Geometry check sheet. Reference: the model listing, model coordinates, mm. A direction names the side the tool comes from. Coordinates: 2 decimals unless noted, no trailing zeros. Write each loop counter-clockwise with the first axis right and the second up, starting at its lowest first coordinate (ties: lowest second). Pieces come first, ordered by that corner, then holes. Notation, with made-up numbers: (-15.5, 70) -> (42.5, 70) arc R10 ccw to (42.5, 86) -> close; hole circle Ø3 at (-2.5, 54). An arc over 180 degrees is marked (long way). Answer in a Markdown table with one row per item. Add a question column.
1. Cross-section at C-C on x = -197. Record the cut outline in (y, z).
2. Cross-section at A-A on y = 122.5. Record the cut outline in (x, z), and give its area (3 significant figures).
3. Cross-section at D-D on x = 57. Record the cut outline in (y, z).
4. Cross-section at B-B on z = 27.5. Record the cut outline in (x, y).
5. Depth check by flat-ended pin: P1, Ø1, axis at x = 134, z = 7, coming from the +Y side; P2, Ø3, axis at x = 190.5, z = 4.5, coming from the +Y side. Enter the tip coordinate at first touch or a pass-through.
6. Mould release check, pull along X, two halves, no side actions. Record for faces 1 (the flat face through (256.851, 121, 19)), 2 (the flat face through (153.663, 242, 19)), 3 (the flat face through (49, 66, 38.1)): pulls with the +X half, pulls with the -X half, needs draft (parallel to the pull), parting line crosses it, or undercut.
7. Scan lines: L1, parallel to X at y = 281.5, z = 8; L2, parallel to Z at x = -175.5, y = 334; L3, parallel to Y at x = 118, z = 34. Record each from-to range of solid material in increasing order. Write a range as from..to.
8. Set-up check for faces 4 (the flat face through (92, 79.238, 19)), 5 (the flat face through (205, 348, 6.35)), 6 (the cylindrical face through (-6.059, 31.626, 19.317)): record each of +Z, -Z, +X, -X, +Y, -Y from which the full face is reachable in a straight line by a thin tool's end or side.
```python
from build123d import *

# Parameters (mm, degrees)
F0_W     = 523.875
F0_H     = 568.325
F1_DEPTH = 38.1
F2_R     = 38.1
F3_DEPTH = 50.8
F4_W     = 317.5
F4_H     = 330.2
F5_DEPTH = 50.8
F6_W     = 896.055773
F6_H     = 120.65
F7_DEPTH = 6.35


with BuildPart() as f1:
    # F0 (on Top) → F1 (new body)
    with BuildSketch(Plane.XY):
        with Locations((-5.086774, 125.275676)):
            Rectangle(F0_W, F0_H)
    extrude(amount=F1_DEPTH)

    # F2 (on face) → F3 (cut)
    with BuildSketch(Plane.XY.offset(38.1)):
        with Locations((-5.086774, 69.713176)):
            Circle(F2_R)
    extrude(amount=-F3_DEPTH, mode=Mode.SUBTRACT)

    # F4 (on face) → F5 (cut)
    with BuildSketch(Plane.XY.offset(38.1)):
        with Locations((-5.086774, 244.338176)):
            Rectangle(F4_W, F4_H)
    extrude(amount=-F5_DEPTH, mode=Mode.SUBTRACT)

    # F6 (on face) → F7 (cut)
    with BuildSketch(Plane(origin=(0, 0, 0), x_dir=(1, 0, 0), z_dir=(0, 0, -1))):
        with Locations((-18.784851, -349.113176)):
            Rectangle(F6_W, F6_H)
    extrude(amount=-F7_DEPTH, mode=Mode.SUBTRACT)


solid = f1.part
```
Results found:
| question | item | result |
|---|---|---|
| 1 | outline | (-158.89, 0) -> (288.79, 0) -> (288.79, 6.35) -> (409.44, 6.35) -> (409.44, 38.1) -> (-158.89, 38.1) -> close |
| 2 | outline | (-267.02, 0) -> (-163.84, 0) -> (-163.84, 38.1) -> (-267.02, 38.1) -> close; (153.66, 0) -> (256.85, 0) -> (256.85, 38.1) -> (153.66, 38.1) -> close |
| 2 | area | 7,860 mm^2 |
| 3 | outline | (-158.89, 0) -> (79.24, 0) -> (79.24, 38.1) -> (-158.89, 38.1) -> close |
| 4 | outline | (-267.02, -158.89) -> (256.85, -158.89) -> (256.85, 409.44) -> (153.66, 409.44) -> (153.66, 79.24) -> (31.8, 79.24) arc R38.1 cw (long way) to (-41.98, 79.24) -> (-163.84, 79.24) -> (-163.84, 409.44) -> (-267.02, 409.44) -> close |
| 5 | P1 | stops at y = 79.24 |
| 5 | P2 | stops at y = 288.79 |
| 6 | face 1 | pulls with the +X half |
| 6 | face 2 | undercut |
| 6 | face 3 | needs draft |
| 7 | L1 | x = -267.02..-163.84, 153.66..256.85 |
| 7 | L2 | z = 6.35..38.1 |
| 7 | L3 | y = -158.89..79.24 |
| 8 | face 4 | +Z, -Z, +Y |
| 8 | face 5 | -Z, +X, -X, +Y |
| 8 | face 6 | +Z, -Z |
